from build123d import *

# Parameters (mm, degrees)
SKETCH1_W           = 30
SKETCH1_H           = 60
SKETCH1_R           = 2.5
BOSS_EXTRUDE1_DEPTH = 1.5
BOSS_EXTRUDE2_START = -20
SKETCH3_R           = 1.5
BOSS_EXTRUDE2_DEPTH = 20
FILLET2_R           = 1
CHAMFER2_SIZE       = 0.5


with BuildPart() as part:
    # Sketch1 → Boss-Extrude1 (new, symmetric)
    with BuildSketch(Plane(origin=(0, 0, 0), x_dir=(0, 0, -1), z_dir=(1, 0, 0))):
        Rectangle(SKETCH1_W, SKETCH1_H)
        with Locations((-7.5, 20)):
            Circle(SKETCH1_R, mode=Mode.SUBTRACT)
        with Locations((7.5, 0)):
            Circle(SKETCH1_R, mode=Mode.SUBTRACT)
        with Locations((-7.5, -20)):
            Circle(SKETCH1_R, mode=Mode.SUBTRACT)
    extrude(amount=BOSS_EXTRUDE1_DEPTH, both=True)

    # Sketch3 → Boss-Extrude2 (add)
    with BuildSketch(Plane(origin=(0, 30, 0), x_dir=(1, 0, 0), z_dir=(0, 1, 0)).offset(BOSS_EXTRUDE2_START)):
        with BuildLine():
            Line((-1.5, -15), (1.5, -15))
            ThreePointArc((1.5, -15), (0, -19.5), (-1.5, -15))
        make_face()
        with Locations(Location((0, -17, 0), (0, 0, 270))):
            Circle(SKETCH3_R, mode=Mode.SUBTRACT)
    extrude(amount=-BOSS_EXTRUDE2_DEPTH)

    # Fillet2
    fillet2_edges = [part.edges().sort_by_distance(p)[0] for p in [
        (1.5, 0, 15),
        (-1.5, 0, 15),
    ]]
    fillet(fillet2_edges, radius=FILLET2_R)

    # Chamfer2
    chamfer2_edges = [part.edges().sort_by_distance(p)[0] for p in [
        (1.5, 0, -15),
        (1.5, 30, 0),
        (-1.5, 30, 0),
        (-1.5, 0, -15),
        (-1.5, -30, 0),
        (1.5, -30, 0),
        (0, 30, 15),
        (0, 30, -15),
        (0, -30, -15),
        (0, -30, 15),
    ]]
    chamfer(chamfer2_edges, length=CHAMFER2_SIZE)


solid = part.part
Could you check a few things on this model? Use its own coordinates, in mm. A direction names the side the tool comes from. Coordinates: 2 decimals unless noted, no trailing zeros. Write each loop counter-clockwise with the first axis right and the second up, starting at its lowest first coordinate (ties: lowest second). Pieces come first, ordered by that corner, then holes. Notation, with made-up numbers: (-9.5, 39) - (17.5, 39) arc R18 ccw to (17.5, 60) - close; hole circle Ø8 at (12, 56). An arc over 180 degrees is marked (long way). Put each result on its own line as item: value. Start each with the question number.
Q1. Which directions (+Z, -Z, +X, -X, +Y, -Y) give clear straight access to the entire face, cutting with the end or side of a thin tool? Please do faces 1 (the cylindrical face through (0.1, 0.1, 19.5)), 2 (the flat face through (0, 20, 15)), 3 (the flat face through (0, -20, 15)).
Q2. Please list where these lines run through material, in increasing order: L1, parallel to Y at x = 0.15, z = 7.5; L2, parallel to X at y = 0.75, z = 17; L3, parallel to Y at x = -0.4, z = -7.5.
Q3. Thinking about a two-plate mould opening in Z: for faces 4 (the cylindrical face through (-0.02, 22.48, 7.83)), 5 (the flat face through (0, 0, -15)), 6 (the flat face through (-1.5, 0, 0)), which applies, pulls with the +Z half, pulls with the -Z half, needs draft (parallel to the pull), parting line crosses it, or undercut?
Q4. I want a section at D-D on y = 4.5. Write out the boundary of the cut face in (x, z).
Q5. I'm going to push flat-ended pins straight in: P1, Ø3, axis at y = -20, z = 7.5, coming from the +X side (3 decimals); P2, Ø1.5, axis at y = 10, z = 6.5, coming from the +X side; P3, Ø10, axis at y = -19, z = 3, coming from the -X side; P4, Ø1.5, axis at x = 1, z = 18, coming from the +Y side. Where does each tip first touch, or does it pass through?
Q6. I want a section at B-B on z = -7.5. Write out the boundary of the cut face in (x, y).
Q7. I want a section at A-A on y = 20. Write out the boundary of the cut face in (x, z), plus the area to 4 significant figures.
Q8. I want a section at C-C on z = -2. Write out the boundary of the cut face in (x, y), plus the area to 4 significant figures.
Checks:
1. face 1: +Y, -Y
1. face 2: +Z, +X, -X, +Y
1. face 3: +Z, +X, -X, -Y
2. L1: -30 to -22.5, -17.5 to 17.5, 22.5 to 30
2. L2: -2.5 to -1.5, 1.5 to 2.5
2. L3: -30 to -2.5, 2.5 to 30
3. face 4: undercut
3. face 5: pulls with the -Z half
3. face 6: needs draft
4. outline: (-1.79, 15.25) arc R1 cw to (-1.5, 14.55) - (-1.5, -14.5) - (-1, -15) - (1, -15) - (1.5, -14.5) - (1.5, 14.55) arc R1 cw to (1.79, 15.25) arc R2.5 ccw (long way) to start; hole circle Ø3 at (0, 17)
5. P1: through
5. P2: x = 1.5
5. P3: x = -1.5
5. P4: y = 10
6. outline: (-1.5, -29.5) - (-1, -30) - (1, -30) - (1.5, -29.5) - (1.5, -2.5) - (-1.5, -2.5) - close; (-1.5, 2.5) - (1.5, 2.5) - (1.5, 29.5) - (1, 30) - (-1, 30) - (-1.5, 29.5) - close
7. outline: (-1.5, -14.5) - (-1, -15) - (1, -15) - (1.5, -14.5) - (1.5, 5) - (-1.5, 5) - close; (-1.5, 10) - (1.5, 10) - (1.5, 15) - (-1.5, 15) - close
7. area: 74.75 mm²
8. outline: (-1.5, -29.5) - (-1, -30) - (1, -30) - (1.5, -29.5) - (1.5, 29.5) - (1, 30) - (-1, 30) - (-1.5, 29.5) - close
8. area: 179.5 mm²
